from build123d import *

# Parameters (mm, degrees)
BOSS_EXTRUDE1_DEPTH = 24
SKETCH2_W           = 24
SKETCH2_H           = 24
BOSS_EXTRUDE2_DEPTH = 16
FILLET1_R           = 12
FILLET2_R           = 12
SKETCH3_W           = 18.1
SKETCH3_H           = 18.1
CUT_EXTRUDE1_DEPTH  = 37
SKETCH4_W           = 18.1
SKETCH4_H           = 18.1
CUT_EXTRUDE2_DEPTH  = 37
SKETCH5_W           = 18.1
SKETCH5_H           = 18.1
CUT_EXTRUDE3_DEPTH  = 37
CHAMFER1_SIZE       = 1


with BuildPart() as part:
    # Sketch1 → Boss-Extrude1 (new body)
    with BuildSketch(Plane(origin=(0, 0, 0), x_dir=(1, 0, 0), z_dir=(0, 1, 0))):
        Polygon((-12, 28), (-12, -12), (28, -12), (28, 12), (12, 12), (12, 28), align=None)
    extrude(amount=BOSS_EXTRUDE1_DEPTH)

    # Sketch2 → Boss-Extrude2 (add)
    with BuildSketch(Plane(origin=(0, 24, 0), x_dir=(1, 0, 0), z_dir=(0, 1, 0))):
        Rectangle(SKETCH2_W, SKETCH2_H)
    extrude(amount=BOSS_EXTRUDE2_DEPTH)

    # Fillet1
    # the kernel refuses this fillet: 12 mm, written as the material it adds along each edge
    with BuildSketch(Plane(origin=(12, 24, 12), x_dir=(1, 0, 0), z_dir=(0, 0, -1))) as fillet1_piece_1:
        with BuildLine():
            CenterArc((FILLET1_R, -FILLET1_R), FILLET1_R, 90, 90)
            Line((0, -FILLET1_R), (0, 0))
            Line((0, 0), (FILLET1_R, 0))
        make_face()
    extrude(amount=24)

    # Fillet2
    # the kernel refuses this fillet: 12 mm, written as the material it adds along each edge
    with BuildSketch(Plane(origin=(12, 0, -12), x_dir=(1, 0, 0), z_dir=(0, 1, 0)), Plane(origin=(12, 24, -12), x_dir=(0, 1, 0), z_dir=(-1, 0, 0))) as fillet2_piece_1:
        with BuildLine():
            CenterArc((FILLET2_R, FILLET2_R), FILLET2_R, 180, 90)
            Line((0, FILLET2_R), (0, 0))
            Line((0, 0), (FILLET2_R, 0))
        make_face()
    extrude(amount=24)
    with BuildSketch(Plane(origin=(42, 24, -12), x_dir=(0, 1, 0), z_dir=(-1, 0, 0))) as fillet2_piece_2a_section:
        with BuildLine():
            CenterArc((FILLET2_R, FILLET2_R), FILLET2_R, 180, 90)
            Line((0, FILLET2_R), (0, 0))
            Line((0, 0), (FILLET2_R, 0))
        make_face()
    fillet2_piece_2a = extrude(amount=54, mode=Mode.PRIVATE)
    fillet2_piece_2a = fillet2_piece_2a - Plane(origin=(24, 36, -15.874937315), x_dir=(1, 0, 0), z_dir=(0, 0, 1)) * Cylinder(12, 156, mode=Mode.PRIVATE)
    fillet2_piece_2a = split(fillet2_piece_2a, bisect_by=Plane(origin=(28, 25.203397989, -15.874937315), z_dir=(-1, 0, 0)), keep=Keep.TOP, mode=Mode.PRIVATE)
    fillet2_piece_2a = split(fillet2_piece_2a, bisect_by=Plane(origin=(12, 25.203397989, -15.874937315), z_dir=(1, 0, 0)), keep=Keep.TOP, mode=Mode.PRIVATE)
    with BuildSketch(Plane(origin=(12, 0, -12), x_dir=(1, 0, 0), z_dir=(0, 1, 0))) as fillet2_piece_2b_section:
        with BuildLine():
            CenterArc((FILLET2_R, FILLET2_R), FILLET2_R, 180, 90)
            Line((0, FILLET2_R), (0, 0))
            Line((0, 0), (FILLET2_R, 0))
        make_face()
    fillet2_piece_2b = extrude(amount=54, mode=Mode.PRIVATE)
    fillet2_piece_2b = fillet2_piece_2b - Plane(origin=(24, 36, -15.874937326), x_dir=(1, 0, 0), z_dir=(0, 0, 1)) * Cylinder(12, 156, mode=Mode.PRIVATE)
    fillet2_piece_2b = split(fillet2_piece_2b, bisect_by=Plane(origin=(13.203398, 24, -15.874937326), z_dir=(0, 1, 0)), keep=Keep.TOP, mode=Mode.PRIVATE)
    fillet2_piece_2b = split(fillet2_piece_2b, bisect_by=Plane(origin=(13.203398, 40, -15.874937326), z_dir=(0, -1, 0)), keep=Keep.TOP, mode=Mode.PRIVATE)
    fillet2_piece_2 = fillet2_piece_2a & fillet2_piece_2b
    add(fillet2_piece_2)

    # Sketch3 → Cut-Extrude1 (cut)
    with BuildSketch(Plane(origin=(28, 0, 0), x_dir=(0, 0, -1), z_dir=(1, 0, 0))):
        with Locations((0.05, 12.05)):
            Rectangle(SKETCH3_W, SKETCH3_H)
    extrude(amount=-CUT_EXTRUDE1_DEPTH, mode=Mode.SUBTRACT)

    # Sketch4 → Cut-Extrude2 (cut)
    with BuildSketch(Plane(origin=(0, 40, 0), x_dir=(1, 0, 0), z_dir=(0, 1, 0))):
        with Locations((0.05, 0.05)):
            Rectangle(SKETCH4_W, SKETCH4_H)
    extrude(amount=-CUT_EXTRUDE2_DEPTH, mode=Mode.SUBTRACT)

    # Sketch5 → Cut-Extrude3 (cut)
    with BuildSketch(Plane(origin=(0, 0, -28), x_dir=(-1, 0, 0), z_dir=(0, 0, -1))):
        with Locations((-0.05, 12.05)):
            Rectangle(SKETCH5_W, SKETCH5_H)
    extrude(amount=-CUT_EXTRUDE3_DEPTH, mode=Mode.SUBTRACT)

    # Chamfer1
    chamfer1_edges = [part.edges().sort_by_distance(p)[0] for p in [
        (12, 12, -28),
        (28, 12, -12),
        (28, 12, 12),
        (-12, 20, 12),
        (-12, 12, -28),
        (28, 24, 0),
        (-12, 38, -12),
        (12, 38, 12),
        (-12, 40, 0),
        (0, 40, 12),
        (12, 40, 0),
        (0, 40, -12),
        (26, 24, 12),
        (15.514718626, 27.514718626, 12),
        (0, 24, -28),
        (12, 0, -26),
        (15.514718626, 0, -15.514718626),
        (-12, 27.514718626, -15.514718626),
        (28, 12.05, -9.1),
        (28, 21.1, -0.05),
        (28, 12.05, 9),
        (28, 3, -0.05),
        (26, 0, -12),
        (28, 0, 0),
        (-12, 24, -26),
        (8, 0, 12),
        (9.1, 40, -0.05),
        (0.05, 40, -9.1),
        (-9, 40, -0.05),
        (0.05, 40, 9),
        (-12, 0, -8),
        (0, 0, -28),
        (-9, 12.05, -28),
        (0.05, 21.1, -28),
        (9.1, 12.05, -28),
        (0.05, 3, -28),
    ]]
    chamfer(chamfer1_edges, length=CHAMFER1_SIZE)


solid = part.part
Design review of the part built by this model. Coordinates are the model's own, in mm. A direction names the side the tool comes from. Give positions to 0.01 mm unless a question says otherwise; leave off trailing zeros. Loops run counter-clockwise (first coordinate to the right, second up) from the corner with the lowest first, then second, coordinate; pieces in that order, holes last. Notation, with made-up numbers: (43.25, -14.75) - (101.25, -14.75) arc R11 ccw to (101.25, -7.75) - close; hole circle Ø8 at (-26, 88.5). An arc over 180 degrees is marked (long way). Write item = value, one per line.
1) Take a section at B-B on y = 4. State the section outline as (x, z) points.
Result sheet:
outline = (-12, -27) - (-11, -28) - (-10, -28) - (-9, -27) - (-9, 9) - (27, 9) - (28, 10) - (28, 11) - (27, 12) - (-11, 12) - (-12, 11) - close; (9.1, -27) - (10.1, -28) - (11, -28) - (12, -27) - (12, -24) arc R12 cw to (24, -12) - (27, -12) - (28, -11) - (28, -10.1) - (27, -9.1) - (9.1, -9.1) - close
2) To check wall thickness, follow line 1 (Z direction, x = 5.5, y = 37.5); line 2 (Y direction, x = 23.5, z = 7); line 3 (X direction, y = 13, z = -23.5). State the ranges of each line that lie inside material, in increasing order.
Result sheet:
line_1 = -12 to -9.1, 9 to 12
line_2 = 0 to 3, 21.1 to 24.01
line_3 = -12 to -9, 9.1 to 12.01
3) Take a section at A-A on z = 4.5. State the section outline as (x, y) points.
Result sheet:
outline = (-12, 1) - (-11, 0) - (27, 0) - (28, 1) - (28, 2) - (27, 3) - (-9, 3) - (-9, 39) - (-10, 40) - (-11, 40) - (-12, 39) - close; (9.1, 21.1) - (27, 21.1) - (28, 22.1) - (28, 23) - (27, 24) - (24, 24) arc R12 cw to (12, 36) - (12, 39) - (11, 40) - (10.1, 40) - (9.1, 39) - close
4) Draft analysis for pull direction X (two halves, no side actions). For faces 1 (the face through (0.9, 22.5, -28)), 2 (the face through (5, 17, 9)), 3 (the face through (5, 3, -5)), 4 (the face through (28, 22.5, 0.9)), state which applies: +X half, -X half, draft (parallel to the pull), parting line (faces both ways), or undercut.
Result sheet:
face_1 = draft
face_2 = undercut
face_3 = undercut
face_4 = +X half
5) Clearance check with flat-ended pins moving along their axes: pin 1 Ø2.5 at (x, z) = (0.5, -25.5) entering from +Y; pin 2 Ø5 at (y, z) = (26, -16.5) entering from +X; pin 3 Ø3 at (y, z) = (18.5, -3) entering from +X. State where each tip first meets the part, or that it passes through.
Result sheet:
pin_1 = 24
pin_2 = 17.37
pin_3 = -9
6) Tool access review of faces 5 (the face through (18, 12, -9.1)), 6 (the face through (1, 37, -12)), 7 (the face through (0, 30, -9.1)), 8 (the face through (26, 12, -12)): name each direction out of +Z, -Z, +X, -X, +Y, -Y from which nothing blocks a thin tool from reaching the whole face with its end or side.
Result sheet:
face_5 = +X
face_6 = -Z, +X, -X, +Y
face_7 = +Y
face_8 = -Z, +X, +Y, -Y
